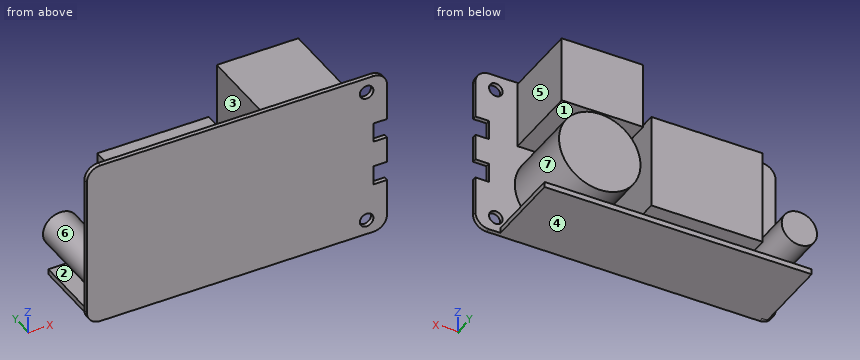
from build123d import *

# Parameters (mm, degrees)
EXTRUDE_1_DEPTH     = 1.6
SKETCH_2_R          = 2.5
CUT_EXTRUDE_1_DEPTH = 1.6
SKETCH_3_R          = 15
SKETCH_3_R_2        = 6.5
SKETCH_3_W          = 98.3
SKETCH_3_H          = 2
SKETCH_3_W_2        = 30
SKETCH_3_H_2        = 24.5
SKETCH_3_W_3        = 41
SKETCH_3_H_3        = 35
EXTRUDE_2_DEPTH     = 29


with BuildPart() as part:
    # 草图1 → 凸台-拉伸1 (new body)
    with BuildSketch(Plane(origin=(0, 0, 0), x_dir=(1, 0, 0), z_dir=(0, 1, 0))):
        with BuildLine():
            Line((55.25, 12.05), (50.25, 12.05))
            Line((50.25, 12.05), (50.25, 4.85))
            Line((50.25, 4.85), (55.25, 4.85))
            Line((55.25, 4.85), (55.25, -4.85))
            Line((55.25, -4.85), (50.25, -4.85))
            Line((50.25, -4.85), (50.25, -12.05))
            Line((50.25, -12.05), (55.25, -12.05))
            Line((55.25, -12.05), (55.25, -25.75))
            ThreePointArc((55.25, -25.75), (53.785533906, -29.285533906), (50.25, -30.75))
            Line((50.25, -30.75), (-50.25, -30.75))
            ThreePointArc((-50.25, -30.75), (-53.785533906, -29.285533906), (-55.25, -25.75))
            Line((-55.25, -25.75), (-55.25, 25.75))
            ThreePointArc((-55.25, 25.75), (-53.785533906, 29.285533906), (-50.25, 30.75))
            Line((-50.25, 30.75), (50.25, 30.75))
            ThreePointArc((50.25, 30.75), (53.785533906, 29.285533906), (55.25, 25.75))
            Line((55.25, 25.75), (55.25, 12.05))
        make_face()
    extrude(amount=EXTRUDE_1_DEPTH)

    # 草图2 → 切除-拉伸1 (cut)
    with BuildSketch(Plane(origin=(0, 1.6, 0), x_dir=(1, 0, 0), z_dir=(0, 1, 0))):
        with Locations((47.75, 25.25)):
            Circle(SKETCH_2_R)
        with Locations((47.75, -25.25)):
            Circle(SKETCH_2_R)
    extrude(amount=-CUT_EXTRUDE_1_DEPTH, mode=Mode.SUBTRACT)

    # 草图3 → 凸台-拉伸2 (add)
    with BuildSketch(Plane(origin=(0, 1.6, 0), x_dir=(1, 0, 0), z_dir=(0, 1, 0))):
        with Locations((25.75, 9.75)):
            Circle(SKETCH_3_R)
        with Locations((-47.75, 14.25)):
            Circle(SKETCH_3_R_2)
        with Locations((-3.1, 29.75)):
            Rectangle(SKETCH_3_W, SKETCH_3_H)
        with Locations((24.75, -18)):
            Rectangle(SKETCH_3_W_2, SKETCH_3_H_2)
        with Locations((-13.75, 6.75)):
            Rectangle(SKETCH_3_W_3, SKETCH_3_H_3)
    extrude(amount=EXTRUDE_2_DEPTH)


solid = part.part
Verification items for the finished model (mm, model axes). Face numbers are marked on the shaded views. A direction names the side the tool comes from. Coordinates: 2 decimals unless noted, no trailing zeros. Loops run counter-clockwise (first coordinate to the right, second up) from the corner with the lowest first, then second, coordinate; pieces in that order, holes last. Notation, with made-up numbers: (56, 27.5) -> (66, 27.5) arc R15 cw to (66, 50.5) -> close; hole circle Ø5 at (-9, -35.75). An arc over 180 degrees is marked (long way). Answer as a JSON object with one key per item and string values. Group by question number.
Item 1: Scan lines: probe 1 along Z at (x, y) = (47.75, 1.15); probe 2 along X at (y, z) = (0.45, -25.25); probe 3 along Z at (x, y) = (-6, 10). Record each from-to range of solid material in increasing order.
Item 2: Sectioned sample at A-A on y = 22. Record the boundary of the cut face in (x, z), plus the area to 3 significant figures.
Item 3: Tool access check on the marked faces 1, 2 and 3. Record the directions out of +Z, -Z, +X, -X, +Y, -Y that give a thin tool (end or side, any length) a straight path to the whole face; none if there is none.
Item 4: Sectioned sample at B-B on x = 47.75. Record the boundary of the cut face in (y, z), plus the area to 3 significant figures.
Item 5: Mould release check, pull along X, two halves, no side actions. Record for the marked faces 4, 5, 6 and 7: +X half, -X half, draft (parallel to the pull), parting line (faces both ways), or undercut.
Item 6: Sectioned sample at D-D on z = -14.25. Record the boundary of the cut face in (x, y).
Item 7: Sectioned sample at C-C on x = -47.75. Record the boundary of the cut face in (y, z).
Item 8: Depth check by flat-ended pin: pin 1 (1 mm diameter, centred on x = -17.5, z = 15, fed in from +Y); pin 2 (5 mm diameter, centred on y = 9.5, z = -12.5, fed in from +X); pin 3 (1.3 mm diameter, centred on x = 53.5, y = 0.5, fed in from +Z). Enter the tip coordinate at first touch or a pass-through.
Evaluation:
{
 "1": {"probe 1": "z = -30.75 to -27.75, -22.75 to 22.75, 27.75 to 30.75", "probe 2": "x = -55.25 to 45.25, 50.25 to 55.25", "probe 3": "z = -30.75 to -28.75, -24.25 to 10.75"},
 "2": {"outline": "circle Ø13 at (-47.75, -14.25); (-52.25, -30.75) -> (46.05, -30.75) -> (46.05, -28.75) -> (-52.25, -28.75) -> close; (-34.25, -24.25) -> (6.75, -24.25) -> (6.75, 10.75) -> (-34.25, 10.75) -> close; (9.75, 5.75) -> (39.75, 5.75) -> (39.75, 30.25) -> (9.75, 30.25) -> close; circle Ø30 at (25.75, -9.75)", "area": "3,210 mm²"},
 "3": {"face 1": "+X, +Y", "face 2": "+X, -X, +Y", "face 3": "+Z, +Y"},
 "4": {"outline": "(0, -30.75) -> (1.6, -30.75) -> (1.6, -27.75) -> (0, -27.75) -> close; (0, -22.75) -> (1.6, -22.75) -> (1.6, 22.75) -> (0, 22.75) -> close; (0, 27.75) -> (1.6, 27.75) -> (1.6, 30.75) -> (0, 30.75) -> close", "area": "82.4 mm²"},
 "5": {"face 4": "draft", "face 5": "+X half", "face 6": "undercut", "face 7": "undercut"},
 "6": {"outline": "(-55.25, 0) -> (55.25, 0) -> (55.25, 1.6) -> (40.06, 1.6) -> (40.06, 30.6) -> (11.44, 30.6) -> (11.44, 1.6) -> (6.75, 1.6) -> (6.75, 30.6) -> (-34.25, 30.6) -> (-34.25, 1.6) -> (-41.25, 1.6) -> (-41.25, 30.6) -> (-54.25, 30.6) -> (-54.25, 1.6) -> (-55.25, 1.6) -> close"},
 "7": {"outline": "(0, -30.75) -> (30.6, -30.75) -> (30.6, -28.75) -> (1.6, -28.75) -> (1.6, -20.75) -> (30.6, -20.75) -> (30.6, -7.75) -> (1.6, -7.75) -> (1.6, 30.75) -> (0, 30.75) -> close"},
 "8": {"pin 1": "stops at y = 1.6", "pin 2": "stops at x = 40.75", "pin 3": "stops at z = 30.02"}
}
